from build123d import *

# Parameters (mm, degrees)
SKETCH1_R           = 27.305
BOSS_EXTRUDE1_DEPTH = 76.2
SKETCH1_3_R         = 3.556
BOSS_EXTRUDE2_DEPTH = 38.1


with BuildPart() as part:
    # Sketch1 → Boss-Extrude1 (new body)
    with BuildSketch(Plane(origin=(0, 0, 0), x_dir=(1, 0, 0), z_dir=(0, 1, 0))):
        with BuildLine():
            Line((26.553308473, 75.046691527), (-24.246691527, 24.246691527))
            ThreePointArc((-24.246691527, 24.246691527), (-31.67982917, -13.122214896), (0, -34.29))
            Line((0, -34.29), (101.6, -34.29))
            ThreePointArc((101.6, -34.29), (133.27982917, -13.122214896), (125.846691527, 24.246691527))
            Line((125.846691527, 24.246691527), (75.046691527, 75.046691527))
            ThreePointArc((75.046691527, 75.046691527), (50.8, 85.09), (26.553308473, 75.046691527))
        make_face()
        with Locations(Location((101.6, 0, 0), (0, 0, 90))):
            Circle(SKETCH1_R, mode=Mode.SUBTRACT)
        with Locations(Location((0, 0, 0), (0, 0, 90))):
            Circle(SKETCH1_R, mode=Mode.SUBTRACT)
        with Locations(Location((50.8, 50.8, 0), (0, 0, 90))):
            Circle(SKETCH1_R, mode=Mode.SUBTRACT)
    extrude(amount=BOSS_EXTRUDE1_DEPTH)

    # Sketch1<3> → Boss-Extrude2 (add)
    # profile 1 of 4: a face of its own
    with BuildSketch(Plane(origin=(0, 0, 0), x_dir=(1, 0, 0), z_dir=(0, 1, 0))):
        with BuildLine():
            Line((-24.246691527, 24.246691527), (-14.203383054, 34.29))
            Line((-14.203383054, 34.29), (-31.75, 34.29))
            ThreePointArc((-31.75, 34.29), (-36.805629933, 31.782278749), (-37.868154158, 26.23979716))
            ThreePointArc((-37.868154158, 26.23979716), (-35.188658815, 13.241319251), (-34.29, -3e-09))
            ThreePointArc((-34.29, -3e-09), (-31.67982917, 13.122214895), (-24.246691527, 24.246691527))
        make_face()
        with Locations(Location((-31.75, 27.94, 0), (0, 0, 90))):
            Circle(SKETCH1_3_R, mode=Mode.SUBTRACT)
    # profile 2 of 4: a face of its own
    with BuildSketch(Plane(origin=(0, 0, 0), x_dir=(1, 0, 0), z_dir=(0, 1, 0))):
        with BuildLine():
            ThreePointArc((0, -34.29), (-24.246691526, -24.246691528), (-34.29, -3e-09))
            ThreePointArc((-34.29, -3e-09), (-35.188658815, -13.241319254), (-37.868154158, -26.23979716))
            ThreePointArc((-37.868154158, -26.23979716), (-36.805629933, -31.782278749), (-31.75, -34.29))
            Line((-31.75, -34.29), (0, -34.29))
        make_face()
        with Locations(Location((-31.75, -27.94, 0), (0, 0, 90))):
            Circle(SKETCH1_3_R, mode=Mode.SUBTRACT)
    # profile 3 of 4: a face of its own
    with BuildSketch(Plane(origin=(0, 0, 0), x_dir=(1, 0, 0), z_dir=(0, 1, 0))):
        with BuildLine():
            Line((133.35, 34.29), (115.803383054, 34.29))
            Line((115.803383054, 34.29), (125.846691527, 24.246691527))
            ThreePointArc((125.846691527, 24.246691527), (133.279829151, 13.122214941), (135.89, 9.8e-08))
            ThreePointArc((135.89, 9.8e-08), (136.788658821, 13.241319301), (139.468154158, 26.23979716))
            ThreePointArc((139.468154158, 26.23979716), (138.405629933, 31.782278749), (133.35, 34.29))
        make_face()
        with Locations(Location((133.35, 27.94, 0), (0, 0, 90))):
            Circle(SKETCH1_3_R, mode=Mode.SUBTRACT)
    # profile 4 of 4: a face of its own
    with BuildSketch(Plane(origin=(0, 0, 0), x_dir=(1, 0, 0), z_dir=(0, 1, 0))):
        with BuildLine():
            ThreePointArc((135.89, 9.8e-08), (125.846691562, -24.246691492), (101.6, -34.29))
            Line((101.6, -34.29), (133.35, -34.29))
            ThreePointArc((133.35, -34.29), (138.405629933, -31.782278749), (139.468154158, -26.23979716))
            ThreePointArc((139.468154158, -26.23979716), (136.788658808, -13.241319204), (135.89, 9.8e-08))
        make_face()
        with Locations(Location((133.35, -27.94, 0), (0, 0, 90))):
            Circle(SKETCH1_3_R, mode=Mode.SUBTRACT)
    extrude(amount=BOSS_EXTRUDE2_DEPTH)


solid = part.part
The listing builds one solid part. Answer for the finished solid, in the listing's coordinates (mm). A direction names the side the tool comes from. Coordinates: 2 decimals unless noted, no trailing zeros. Order: outer loops, then holes, each group sorted by start corner. A loop starts at its lowest first (then second) coordinate and runs counter-clockwise, first axis right, second up.
Q1. A cutting plane is placed at C-C, the plane y = 19.5. Write down the section's boundary in (x, z) (3 decimals).
Q2. Which of the six approach directions +Z, -Z, +X, -X, +Y, -Y give full straight-line access (tool end or side, diameter ignored) to faces 5 (the face through (-23, 19, -34.29)), 6 (the face through (130, 38.1, -25)), 7 (the face through (125, 19, -34.29))?
Q3. Given P1, Ø9, axis at x = -19, y = 22.5, coming from the -Z side; P2, Ø8, axis at x = 133.35, z = 27.94, coming from the -Y side; P3, Ø8, axis at x = 58, y = 44.5, coming from the -Z side; P4, Ø12, axis at x = 78, y = 10, coming from the -Z side, each flat-ended and moving along its own axis, determine where each tip first touches the part or whether it passes through.
Q4. A cutting plane is placed at B-B, the plane y = 61. Write down the section's boundary in (x, z) (3 decimals).
Q5. A cutting plane is placed at A-A, the plane x = 50.8. Write down the section's boundary in (y, z) (3 decimals).
Q6. A cutting plane is placed at D-D, the plane z = -41. Write down the section's boundary in (x, y), and give its area (3 significant figures).
Q7. Consider line 1 (X direction, y = 17.5, z = 27.94); line 2 (X direction, y = 26, z = -8); line 3 (X direction, y = 19, z = -27.94). Determine where each line is inside the solid, lowest interval first.
Q8. For a pull along Z with two mould halves and no side action, classify faces 1 (the face through (125.824, 37.567, -12.6)), 2 (the face through (129, 38.1, 26)), 3 (the face through (50, 29, 34.29)), 4 (the face through (129.824, 18.783, 28.403)) as pulls with the +Z half, pulls with the -Z half, needs draft (parallel to the pull), parting line crosses it, or undercut.
Answers follow:
1. outline: (-37.868, -26.24) arc R6.35 ccw to (-31.75, -34.29) - (-14.203, -34.29) - (26.553, -75.047) arc R34.29 ccw to (75.047, -75.047) - (115.803, -34.29) - (133.35, -34.29) arc R6.35 ccw to (139.468, -26.24) arc R98.002 cw to (139.468, 26.24) arc R6.35 ccw to (133.35, 34.29) - (-31.75, 34.29) arc R6.35 ccw to (-37.868, 26.24) arc R98.002 cw to start; hole circle Ø7.112 at (-31.75, -27.94); hole circle Ø7.112 at (-31.75, 27.94); hole circle Ø54.61 at (0, 0); hole circle Ø54.61 at (50.8, -50.8); hole circle Ø54.61 at (101.6, 0); hole circle Ø7.112 at (133.35, -27.94); hole circle Ø7.112 at (133.35, 27.94)
2. face 5: -Z, -X, +Y, -Y
2. face 6: -Z, +X, +Y
2. face 7: -Z, +X, +Y, -Y
3. P1: stops at z = -34.29
3. P2: stops at y = 0
3. P3: stops at z = -84.94
3. P4: stops at z = -77.75
4. outline: (-24.247, -24.247) - (26.553, -75.047) arc R34.29 ccw to (75.047, -75.047) - (125.847, -24.247) arc R34.29 ccw to (101.6, 34.29) - (0, 34.29) arc R34.29 ccw to start; hole circle Ø54.61 at (0, 0); hole circle Ø54.61 at (50.8, -50.8); hole circle Ø54.61 at (101.6, 0)
5. outline: (0, -85.09) - (76.2, -85.09) - (76.2, -78.105) - (0, -78.105) - close; (0, -23.495) - (76.2, -23.495) - (76.2, 34.29) - (0, 34.29) - close
6. outline: (-7.49, 0) - (25.31, 0) - (25.31, 76.2) - (-7.49, 76.2) - close; (76.29, 0) - (109.09, 0) - (109.09, 76.2) - (76.29, 76.2) - close
6. area: 5,000 mm2
7. line 1: x = -38.1 to -35.31, -28.19 to 129.79, 136.91 to 139.7
7. line 2: x = -34.62 to -26.11, 26.11 to 75.49, 127.71 to 136.22
7. line 3: x = -38.1 to -35.31, -28.19 to 35.87, 65.73 to 129.79, 136.91 to 139.7
8. face 1: undercut
8. face 2: needs draft
8. face 3: pulls with the +Z half
8. face 4: undercut
